Geometry check sheet. Reference: the model listing, model coordinates, mm. Face numbers are marked on the shaded views. A direction names the side the tool comes from. Give positions to 0.01 mm unless a question says otherwise; leave off trailing zeros. Write each loop counter-clockwise with the first axis right and the second up, starting at its lowest first coordinate (ties: lowest second). Pieces come first, ordered by that corner, then holes. Notation, with made-up numbers: M 53.5,-26.5 L 71.5,-26.5 A25 cw 71.5,0.5 Z; hole C 29.25,19 d6. An arc over 180 degrees is marked long. Write each question's results on one line, items separated by ' | '.
```python
from build123d import *

# Parameters (mm, degrees)
SKETCH1_R     = 6.223
SKETCH1_R_2   = 3.175
CHAMFER1_SIZE = 0.5
SKETCH4_W     = 2.0193
SKETCH4_H     = 6.223


with BuildPart() as part:
    # Sweep1: sweep along a path in Sketch2
    with BuildLine(Plane(origin=(0, 0, 0), x_dir=(1, 0, 0), z_dir=(0, 1, 0))) as sweep1_path:
        Line((0, -3.9878), (0, 3.9878))
    # Sketch1 → Sweep1 (sweep)
    with BuildSketch(Plane.XY):
        Circle(SKETCH1_R)
        Circle(SKETCH1_R_2, mode=Mode.SUBTRACT)
    sweep(path=sweep1_path.line)

    # Chamfer1
    chamfer1_edges = [part.edges().sort_by_distance(p)[0] for p in [
        (-6.223, 0, 3.9878),
        (-6.223, 0, -3.9878),
    ]]
    chamfer(chamfer1_edges, length=CHAMFER1_SIZE)

    # Sketch4 → Tap Drill for #10-32 Tap1 (revolve, cut)
    with BuildSketch(Plane(origin=(0, 0, 0), x_dir=(0, 0, -1), z_dir=(1, 0, 0))):
        with Locations((1.00965, 3.1115)):
            Rectangle(SKETCH4_W, SKETCH4_H)
    revolve(axis=Axis((0, -6.35, 0), (0, 1, 0)), mode=Mode.SUBTRACT)


solid = part.part
```
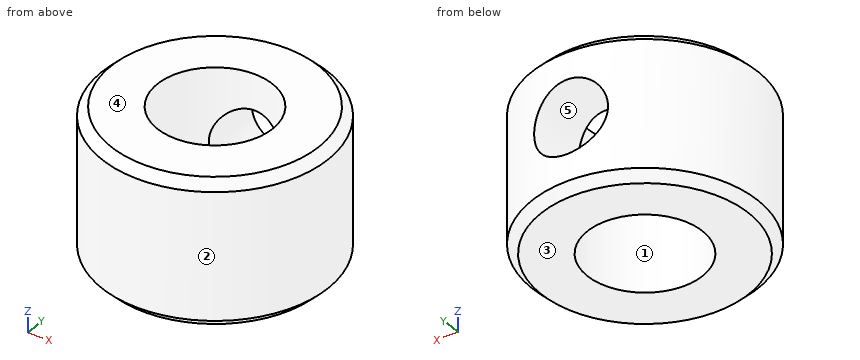
Q1. Depth check by flat-ended pin: P1, Ø3, axis at y = 2.5, z = 3, coming from the -X side; P2, Ø2, axis at x = 3, z = 2, coming from the +Y side; P3, Ø1, axis at x = -4, z = 0.5, coming from the -Y side. Enter the tip coordinate at first touch or a pass-through.
Answer key:
P1: stops at x = -6.14 | P2: stops at y = 5.89 | P3: stops at y = -5.15
Q2. Section check B-B (z = 3). Enter the section's corners in (x, y) (3 decimals), then the cut area to 3 significant figures.
Answer key:
outline: C 0,0 d12.446; hole C 0,0 d6.35 | area: 90.0 mm2
Q3. Section check A-A (y = 0). Enter the section's corners in (x, z) (3 decimals).
Answer key:
outline: M -6.223,-3.488 L -5.723,-3.988 L -3.175,-3.988 L -3.175,3.988 L -5.723,3.988 L -6.223,3.488 Z; M 3.175,-3.988 L 5.723,-3.988 L 6.223,-3.488 L 6.223,3.488 L 5.723,3.988 L 3.175,3.988 Z
Q4. Section check D-D (z = 1.5). Enter the section's corners in (x, y) (3 decimals).
Answer key:
outline: M -1.352,2.873 L -1.352,6.074 A6.223 ccw long 1.352,6.074 L 1.352,2.873 A3.175 cw long Z
Q5. Section check C-C (x = -0.25). State how many separate pieces and enclosed holes the cut face has, then the cut area to 3 significant figures.
Answer key:
separate pieces: 3 | enclosed holes: 0 | area: 36.0 mm2
Q6. Release check for a two-part mould opening along Y. For the marked faces 1, 2 and 3 record: released by +Y, released by -Y, zero draft, split by the parting line, or undercut.
Answer key:
face 1: undercut | face 2: split by the parting line | face 3: zero draft
Q7. Access from +Z, -Z, +X, -X, +Y, -Y to the whole of each face (thin tool, end or side, straight path). Record for the marked faces 4 and 5.
Answer key:
face 4: +Z, +X, -X, +Y, -Y | face 5: +Y
Q8. Material ranges on probe 1 along Y at (x, z) = (0, -2.25) (3 decimals); probe 2 along Z at (x, y) = (0, 4.35); probe 3 along Y at (x, z) = (-2, 3.75), recorded low to high. Write a range as [from, to].
Answer key:
probe 1: y = [-6.223, -3.175], [3.175, 6.223] | probe 2: z = [-3.99, -2.02], [2.02, 3.99] | probe 3: y = [-5.62, -2.47], [2.47, 5.62]
